```python
from build123d import *

# Parameters (mm, degrees)
CYLINDER004_R     = 2
CYLINDER004_DEPTH = 10
BOX003_W          = 8
BOX003_H          = 8
BOX003_DEPTH      = 10
FILLET_R          = 2
CYLINDER005_R     = 2
CYLINDER005_DEPTH = 10
BOX004_W          = 8
BOX004_H          = 8
BOX004_DEPTH      = 10
FILLET001_R       = 2
PAD001_DEPTH      = 5
BOX001_W          = 25.6
BOX001_H          = 16
BOX001_DEPTH      = 10


with BuildPart() as cylinder004:
    # Cylinder004 → Cylinder004 (new body)
    with BuildSketch(Plane(origin=(4, 4, 0), x_dir=(1, 0, 0), z_dir=(0, 0, 1))):
        Circle(CYLINDER004_R)
    extrude(amount=CYLINDER004_DEPTH)


with BuildPart() as fillet_body:
    # Box003 → Box003 (new body)
    with BuildSketch(Plane.XY):
        with Locations((4, 4)):
            Rectangle(BOX003_W, BOX003_H)
    extrude(amount=BOX003_DEPTH)

    # Cut004: cut Cylinder004
    add(cylinder004.part, mode=Mode.SUBTRACT)


with BuildPart() as fillet_body_1:
    # Cut004 placement: moved
    add(fillet_body.part.moved(Location((30, -10, 0))))

    # Fillet
    fillet_edges = [fillet_body_1.edges().sort_by_distance(p)[0] for p in [
        (30, -10, 5),
        (38, -10, 5),
    ]]
    fillet(fillet_edges, radius=FILLET_R)


with BuildPart() as cylinder005:
    # Cylinder005 → Cylinder005 (new body)
    with BuildSketch(Plane(origin=(4, 4, 0), x_dir=(1, 0, 0), z_dir=(0, 0, 1))):
        Circle(CYLINDER005_R)
    extrude(amount=CYLINDER005_DEPTH)


with BuildPart() as fillet001:
    # Box004 → Box004 (new body)
    with BuildSketch(Plane.XY):
        with Locations((4, 4)):
            Rectangle(BOX004_W, BOX004_H)
    extrude(amount=BOX004_DEPTH)

    # Cut005: cut Cylinder005
    add(cylinder005.part, mode=Mode.SUBTRACT)


with BuildPart() as fillet001_1:
    # Cut005 placement: moved
    add(fillet001.part.moved(Location((45, 14, 0))))

    # Fillet001
    fillet001_edges = [fillet001_1.edges().sort_by_distance(p)[0] for p in [
        (45, 22, 5),
        (53, 22, 5),
    ]]
    fillet(fillet001_edges, radius=FILLET001_R)


with BuildPart() as obj1:
    # Sketch001 → Pad001 (new body)
    with BuildSketch(Plane(origin=(0, 0, 0), x_dir=(-1, 0, 0), z_dir=(0, 0, 1))):
        Polygon((-30, 0), (-30, -13), (-55.6, -7.5), (-55.6, 0), align=None)
    extrude(amount=PAD001_DEPTH)


with BuildPart() as obj1_1:
    # Body001 placement: moved
    add(obj1.part.moved(Location((0, 0, 5))))


with BuildPart() as f_200mm:
    # Box001 → Box001 (new body)
    with BuildSketch(Plane(origin=(30, -2, 0), x_dir=(1, 0, 0), z_dir=(0, 0, 1))):
        with Locations((12.8, 8)):
            Rectangle(BOX001_W, BOX001_H)
    extrude(amount=BOX001_DEPTH)

    # Cut001: cut obj1
    add(obj1_1.part, mode=Mode.SUBTRACT)

    # Fusion: union Fillet body, Fillet001
    add(fillet_body_1.part)
    add(fillet001_1.part)


solid = f_200mm.part
```
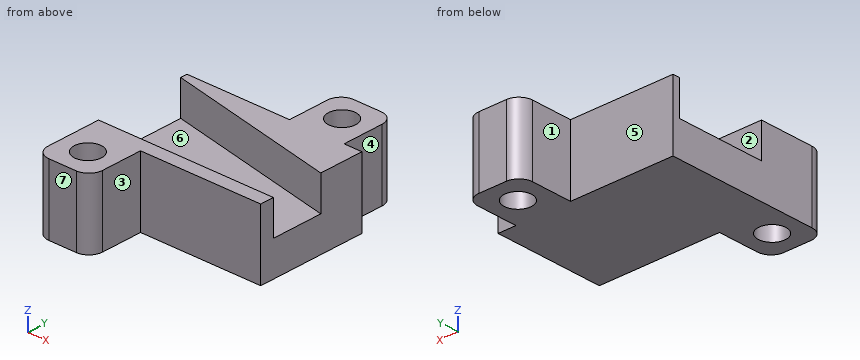
Geometry check sheet. Reference: the model listing, model coordinates, mm. Face numbers are marked on the shaded views. A direction names the side the tool comes from. Coordinates: 2 decimals unless noted, no trailing zeros. Order: outer loops, then holes, each group sorted by start corner. A loop starts at its lowest first (then second) coordinate and runs counter-clockwise, first axis right, second up. Notation, with made-up numbers: M 75.5,80.5 L 100.5,80.5 A15 cw 100.5,109.5 Z; hole C -35.75,-36.75 d1. An arc over 180 degrees is marked long. One line per question, with ' | ' between items. Start each with the question number.
Item 1: Draft check along Y on the marked faces 5, 6 and 7. Enter one of: pulls with the +Y half, pulls with the -Y half, needs draft (parallel to the pull), parting line crosses it, or undercut.
Item 2: Set-up check for the marked faces 1, 2, 3 and 4: record each of +Z, -Z, +X, -X, +Y, -Y from which the full face is reachable in a straight line by a thin tool's end or side.
Item 3: Material ranges on L1, parallel to Y at x = 34, z = 2; L2, parallel to Y at x = 49, z = 6.5; L3, parallel to Y at x = 49, z = 4.75, recorded low to high. Write a range as [from, to].
Item 4: Gauge pin test, flat ends, axial feed: pin 1 (1.3 mm diameter, centred on x = 55, z = 5.5, fed in from +Y); pin 2 (1.5 mm diameter, centred on x = 50.5, z = 9, fed in from -Y); pin 3 (2 mm diameter, centred on x = 43, y = 0, fed in from -Z); pin 4 (2.5 mm diameter, centred on x = 49, y = 18, fed in from +Z). Record the tip position at first contact, or that the pin passes through.
Item 5: Cross-section at C-C on x = 49.25. Enter the section's corners in (y, z), then the cut area to 3 significant figures.
Item 6: Cross-section at B-B on z = 6.25. Enter the section's corners in (x, y), then the cut area to 3 significant figures.
Item 7: Cross-section at D-D on z = 4.25. Enter the section's corners in (x, y), then the cut area to 3 significant figures.
Item 8: Cross-section at A-A on y = -6. Enter the section's corners in (x, z).
Findings:
1) face 5: pulls with the +Y half | face 6: undercut | face 7: pulls with the -Y half
2) face 1: +Z, -Z, -X, +Y | face 2: +Z, +X, -X | face 3: +Z, -Z, +X, -Y | face 4: +Z, -Z, +X, +Y
3) L1: y = [-10, -8], [-4, 14] | L2: y = [-2, 0], [8.92, 16], [20, 22] | L3: y = [-2, 16], [20, 22]
4) pin 1: stops at y = 14 | pin 2: stops at y = -2 | pin 3: stops at z = 0 | pin 4: passes through
5) outline: M -2,0 L 16.02,0 L 16.02,10 L 8.86,10 L 8.86,5 L 0,5 L 0,10 L -2,10 Z; M 19.98,0 L 22,0 L 22,10 L 19.98,10 Z | area: 156 mm²
6) outline: M 30,-8 A2 ccw 32,-10 L 36,-10 A2 ccw 38,-8 L 38,-2 L 55.6,-2 L 55.6,0 L 30,0 Z; M 30,13 L 55.6,7.5 L 55.6,14 L 53,14 L 53,20 A2 ccw 51,22 L 47,22 A2 ccw 45,20 L 45,14 L 30,14 Z; hole C 34,-6 d4; hole C 49,18 d4 | area: 247 mm²
7) outline: M 30,-8 A2 ccw 32,-10 L 36,-10 A2 ccw 38,-8 L 38,-2 L 55.6,-2 L 55.6,14 L 53,14 L 53,20 A2 ccw 51,22 L 47,22 A2 ccw 45,20 L 45,14 L 30,14 Z; hole C 34,-6 d4; hole C 49,18 d4 | area: 509 mm²
8) outline: M 30,0 L 32,0 L 32,10 L 30,10 Z; M 36,0 L 38,0 L 38,10 L 36,10 Z
